```python
from build123d import *

# Parameters (mm, degrees)
BOSS_EXTRUDE1_DEPTH            = 40
SKETCH2_W                      = 40
SKETCH2_H                      = 30
BOSS_EXTRUDE2_DEPTH            = 20
BOSS_EXTRUDE3_DEPTH            = 30
CUT_EXTRUDE1_DEPTH             = 30
SKETCH5_W                      = 70
SKETCH5_H                      = 40
BOSS_EXTRUDE4_DEPTH            = 10
SKETCH6_W                      = 20
SKETCH6_H                      = 20
CUT_EXTRUDE2_DEPTH             = 41
F_10_0_10_DIAMETER_HOLE1_D     = 10
F_10_0_10_DIAMETER_HOLE1_DEPTH = 40
FILLET1_R                      = 20


with BuildPart() as part:
    # Sketch1 → Boss-Extrude1 (new body)
    with BuildSketch(Plane(origin=(0, 0, 0), x_dir=(0, -1, 0), z_dir=(-1, 0, 0))):
        Polygon((-10, -8), (-40, -20), (-10, -20), align=None)
    extrude(amount=-BOSS_EXTRUDE1_DEPTH)

    # Sketch2 → Boss-Extrude2 (add)
    with BuildSketch(Plane(origin=(0, 0, -20), x_dir=(-1, 0, 0), z_dir=(0, 0, -1))):
        with Locations((-20, 25)):
            Rectangle(SKETCH2_W, SKETCH2_H)
    extrude(amount=BOSS_EXTRUDE2_DEPTH)

    # Sketch3 → Boss-Extrude3 (add)
    with BuildSketch(Plane(origin=(40, 0, 0), x_dir=(0, 0, -1), z_dir=(1, 0, 0))):
        Polygon((40, 10), (0, 10), (20, 40), (40, 40), align=None)
    extrude(amount=BOSS_EXTRUDE3_DEPTH)

    # Sketch4 → Cut-Extrude1 (cut)
    with BuildSketch(Plane(origin=(70, 0, 0), x_dir=(0, 0, -1), z_dir=(1, 0, 0))):
        Polygon((20, 40), (0, 10), (30, 10), (30, 30), (40, 30), (40, 40), align=None)
    extrude(amount=-CUT_EXTRUDE1_DEPTH, mode=Mode.SUBTRACT)

    # Sketch5 → Boss-Extrude4 (add)
    with BuildSketch(Plane.XZ.offset(-10)):
        with Locations((35, -20)):
            Rectangle(SKETCH5_W, SKETCH5_H)
    extrude(amount=BOSS_EXTRUDE4_DEPTH)

    # Sketch6 → Cut-Extrude2 (cut, through all)
    with BuildSketch(Plane(origin=(0, 0, -40), x_dir=(-1, 0, 0), z_dir=(0, 0, -1))):
        with Locations((-20, 30)):
            Rectangle(SKETCH6_W, SKETCH6_H)
    extrude(amount=-CUT_EXTRUDE2_DEPTH, mode=Mode.SUBTRACT)

    # Ø10.0 (10) Diameter Hole1
    with Locations(Plane(origin=(0, 0, 0), x_dir=(-1, 0, 0), z_dir=(0, -1, 0))):
        with Locations((-55, 15)):
            Hole(F_10_0_10_DIAMETER_HOLE1_D / 2, depth=F_10_0_10_DIAMETER_HOLE1_DEPTH)

    # Fillet1
    fillet1_edges = [part.edges().sort_by_distance(p)[0] for p in [
        (70, 30, -35),
    ]]
    fillet(fillet1_edges, radius=FILLET1_R)


solid = part.part
```
Check sheet for the modelled part. Datum: model origin and axes. Units: mm. A direction names the side the tool comes from. Coordinates: 2 decimals unless noted, no trailing zeros. Order: outer loops, then holes, each group sorted by start corner. A loop starts at its lowest first (then second) coordinate and runs counter-clockwise, first axis right, second up. Notation, with made-up numbers: M 53.5,57.25 L 83.5,57.25 A32 ccw 83.5,86.25 Z; hole C 45,-19 d9. An arc over 180 degrees is marked long. One line per question, with ' | ' between items. Start each with the question number.
Item 1: Sectioned sample at A-A on y = 32.5. Record the cut outline in (x, z).
Item 2: Material ranges on line 1 (X direction, y = 25, z = -21.5); line 2 (Z direction, x = 31, y = 15); line 3 (Z direction, x = 55, y = 5), recorded low to high.
Item 3: Sectioned sample at B-B on z = -15. Record the cut outline in (x, y), and give its area (3 significant figures).
Item 4: Sectioned sample at C-C on x = 34.5. Record the cut outline in (y, z).
Item 5: Gauge pin test, flat ends, axial feed: P1, Ø5, axis at x = 44, z = -32.5, coming from the +Y side; P2, Ø24, axis at x = 52.5, z = -10.5, coming from the +Y side; P3, Ø24, axis at y = 23.5, z = -21, coming from the +X side; P4, Ø6, axis at x = 55, z = -15, coming from the +Y side. Record the tip position at first contact, or that the pin passes through.
Item 6: Access from +Z, -Z, +X, -X, +Y, -Y to the whole of each face (thin tool, end or side, straight path). Record for faces 1 (the flat face through (42, 10, -11)), 2 (the flat face through (20, 20, -26)), 3 (the flat face through (35, 40, -30)), 4 (the flat face through (45, 30, -35)), 5 (the flat face through (35, 5, 0)).
Item 7: Sectioned sample at D-D on y = 6.5. Record the cut outline in (x, z), and give its area (3 significant figures).
Item 8: Mould release check, pull along X, two halves, no side actions. Record for faces 6 (the flat face through (30, 30, -29)), 7 (the flat face through (35, 16, -40)), 8 (the flat face through (70, 5, -20)): pulls with the +X half, pulls with the -X half, needs draft (parallel to the pull), parting line crosses it, or undercut.
Answer below:
1) outline: M 0,-40 L 10,-40 L 10,-17 L 0,-17 Z; M 30,-40 L 40,-40 L 40,-17 L 30,-17 Z
2) line 1: x = 0 to 10, 30 to 40 | line 2: z = -40 to -10 | line 3: z = -40 to -20, -10 to 0
3) outline: M 0,0 L 50,0 L 50,10 L 40,10 L 40,27.5 L 30,27.5 L 30,20 L 10,20 L 10,27.5 L 0,27.5 Z; M 60,0 L 70,0 L 70,10 L 60,10 Z | area: 1,150 mm^2
4) outline: M 0,-40 L 40,-40 L 40,-20 L 10,-8 L 10,0 L 0,0 Z
5) P1: stops at y = 30 | P2: stops at y = 10 | P3: stops at x = 69.21 | P4: passes through
6) face 1: +Z, +X, +Y | face 2: +Z, -Z, +Y | face 3: +Z, -Z, +X, -X, +Y | face 4: +Z, -Z, +X, +Y | face 5: +Z, +X, -X, +Y, -Y
7) outline: M 0,-40 L 70,-40 L 70,0 L 0,0 Z; hole C 55,-15 d10 | area: 2,720 mm^2
8) face 6: undercut | face 7: needs draft | face 8: pulls with the +X half
